Check sheet for the modelled part. Datum: model origin and axes. Units: mm. Face numbers are marked on the shaded views. A direction names the side the tool comes from. Coordinates: 2 decimals unless noted, no trailing zeros. Write each loop counter-clockwise with the first axis right and the second up, starting at its lowest first coordinate (ties: lowest second). Pieces come first, ordered by that corner, then holes. Notation, with made-up numbers: (-40, 72.5) -> (3, 72.5) arc R28 ccw to (3, 108.5) -> close; hole circle Ø11 at (85, 72). An arc over 180 degrees is marked (long way). One line per item, written item: value. Start each with the question number.
1) Sectioned sample at A-A on z = -88. Enter the section's corners in (x, y).
2) Sectioned sample at B-B on y = -4. Enter the section's corners in (x, z).
3) Set-up check for the marked faces 1, 2 and 3: record each of +Z, -Z, +X, -X, +Y, -Y from which the full face is reachable in a straight line by a thin tool's end or side.
4) Sectioned sample at D-D on y = -16. Enter the section's corners in (x, z).
5) Gauge pin test, flat ends, axial feed: P1, Ø4, axis at x = 48.5, z = -10, coming from the +Y side; P2, Ø9, axis at x = 44.5, y = -10, coming from the -Z side; P3, Ø1.5, axis at x = 31.5, z = -29, coming from the -Y side; P4, Ø9, axis at x = 34.81, z = -8, coming from the +Y side. Record the tip position at first contact, or that the pin passes through.
6) Draft check along Z on the marked faces 4, 5, 6 and 7. Enter one of: +Z half, -Z half, draft (parallel to the pull), parting line (faces both ways), or undercut.
7) Sectioned sample at C-C on z = -34. Enter the section's corners in (x, y).
8) Scan lines: line 1 along Z through (x, y) = (47, -9.5); line 2 along Z through (x, y) = (48, -13.5); line 3 along Z through (x, y) = (34, 7.25). Record each from-to range of solid material in increasing order. Write a range as [from, to].
```python
from build123d import *

# Parameters (mm, degrees)
SKETCH1_W                       = 52.809375
SKETCH1_H                       = 85
BOSS_EXTRUDE1_DEPTH             = 10
SPRING_PULLEY_CUTOUT_DEPTH      = 10
SPRING_PULLEY_CUTOUT_DEPTH_BACK = 11
SKETCH2_R                       = 24
BOSS_EXTRUDE4_DEPTH             = 23
SKETCH20_R                      = 2.75
CUT_EXTRUDE8_DEPTH              = 104.912607935
MOVE_START                      = -18
MOVE_FACE1_OUTLINE_W            = 23
MOVE_FACE1_OUTLINE_H            = 5
MOVE_FACE1_DEPTH                = 18
MOVE_FACE3_BY                   = 1
MOVE_FACE4_BY                   = 0.809375
FILLET4_R                       = 2
BOSS_EXTRUDE5_START             = -10
BOSS_EXTRUDE5_DEPTH             = 10
SKETCH38_R                      = 2.75
CUT_EXTRUDE9_DEPTH              = 118.140215502
CUT_EXTRUDE10_DEPTH             = 5


# Read off the part's stored shape, not the designer's step: Move Face1
with BuildPart() as part:
    # Sketch1 → Boss-Extrude1 (new body)
    with BuildSketch(Plane(origin=(0, 0, 0), x_dir=(1, 0, 0), z_dir=(0, 1, 0))):
        with Locations((26.4046875, 42.5)):
            Rectangle(SKETCH1_W, SKETCH1_H)
    extrude(amount=BOSS_EXTRUDE1_DEPTH)

    # Sketch2 → spring_pulley_cutout (cut, two sides: drawn at the far end of the back side and taken through both)
    with BuildSketch(Plane.ZY.offset(-18).offset(-SPRING_PULLEY_CUTOUT_DEPTH_BACK)):
        with Locations((-34, -18.5)):
            Circle(SKETCH2_R)
    extrude(amount=SPRING_PULLEY_CUTOUT_DEPTH + SPRING_PULLEY_CUTOUT_DEPTH_BACK, mode=Mode.SUBTRACT)

    # Sketch34 → Cut-Revolve1 (revolve, cut)
    with BuildSketch(Plane(origin=(16, 0, 0), x_dir=(0, 0, -1), z_dir=(1, 0, 0))):
        Polygon((16.798424815, -5.423086457), (21.139079438, 10.776457135), (24.036856917, 10), (23.001580737, 6.136296695), (21.069729084, 6.653934785), (17.764350642, -5.681905502), align=None)
    revolve(axis=Axis((16, -5.423086457, -16.798424815), (0, 0.9659258262890682, -0.2588190451025213)), mode=Mode.SUBTRACT)

    # Sketch36 → Cut-Revolve2 (revolve, cut)
    with BuildSketch(Plane(origin=(21, 0, 0), x_dir=(0, 0, -1), z_dir=(1, 0, 0)), mode=Mode.PRIVATE) as cut_revolve2_sk:
        Polygon((50.543888978, -2.968568117), (46.860920562, 10.776457135), (43.963143083, 10), (44.998419263, 6.136296695), (46.930270916, 6.653934785), (49.577963152, -3.227387162), align=None)
    revolve(cut_revolve2_sk.sketch.rotate(Axis((21, -2.968568117, -50.543888978), (0, 0.9659258262890665, 0.2588190451025275)), 180), axis=Axis((21, -2.968568117, -50.543888978), (0, 0.9659258262890665, 0.2588190451025275)), mode=Mode.SUBTRACT)

    # Sketch19 → Boss-Extrude4 (add)
    with BuildSketch(Plane.ZY.offset(-29.809375)):
        with BuildLine():
            Line((-68, -18), (-68, 0))
            Line((-68, 0), (0, 0))
            Line((0, 0), (0, -18))
            Line((0, -18), (-16.006945785, -18))
            ThreePointArc((-16.006945785, -18), (-34, -0.5), (-51.993054215, -18))
            Line((-51.993054215, -18), (-68, -18))
        make_face()
    extrude(amount=-BOSS_EXTRUDE4_DEPTH)

    # Sketch20 → Cut-Extrude8 (cut, through all)
    with BuildSketch(Plane(origin=(0, -18, 0), x_dir=(-1, 0, 0), z_dir=(0, -1, 0))):
        with Locations(Location((-47.809375, 8.003472892, 0), (0, 0, 90))):
            Circle(SKETCH20_R)
        with Locations(Location((-34.809375, 8.003472892, 0), (0, 0, 90))):
            Circle(SKETCH20_R)
        with Locations(Location((-47.809375, 59.996527108, 0), (0, 0, 90))):
            Circle(SKETCH20_R)
        with Locations(Location((-34.809375, 59.996527108, 0), (0, 0, 90))):
            Circle(SKETCH20_R)
    extrude(amount=-CUT_EXTRUDE8_DEPTH, mode=Mode.SUBTRACT)

    # Move Face1 outline → Move Face1 (add)
    with BuildSketch(Plane(origin=(0, 0, 0), x_dir=(1, 0, 0), z_dir=(0, 1, 0)).offset(MOVE_START)):
        with Locations((41.309375, 70.5)):
            Rectangle(MOVE_FACE1_OUTLINE_W, MOVE_FACE1_OUTLINE_H)
    extrude(amount=MOVE_FACE1_DEPTH)

    # Move Face3: a face moved inward by 1.0
    extrude(part.faces().sort_by_distance((8, 2.223147927, -34))[0], amount=MOVE_FACE3_BY, dir=(-1, 0, 0), mode=Mode.SUBTRACT)

    # Move Face4: a face moved inward by 0.809375
    extrude(part.faces().sort_by_distance((29, 2.223147927, -34))[0], amount=MOVE_FACE4_BY, dir=(1, 0, 0), mode=Mode.SUBTRACT)

    # Fillet4
    fillet4_edges = [part.edges().sort_by_distance(p)[0] for p in [
        (52.809375, -9, -73),
        (29.809375, -9, 0),
        (29.809375, -9, -73),
        (0, 5, -85),
        (52.809375, 5, -85),
        (52.809375, -4, 0),
        (0, 5, 0),
    ]]
    fillet(fillet4_edges, radius=FILLET4_R)

    # Sketch37 → Boss-Extrude5 (add)
    with BuildSketch(Plane.XZ.offset(BOSS_EXTRUDE5_START)):
        with BuildLine():
            Line((0, -83), (0, -101))
            ThreePointArc((0, -101), (0.585786438, -102.414213562), (2, -103))
            Line((2, -103), (50.809375, -103))
            ThreePointArc((50.809375, -103), (52.223588562, -102.414213562), (52.809375, -101))
            Line((52.809375, -101), (52.809375, -83))
            ThreePointArc((52.809375, -83), (52.223588562, -84.414213562), (50.809375, -85))
            Line((50.809375, -85), (2, -85))
            ThreePointArc((2, -85), (0.585786438, -84.414213562), (0, -83))
        make_face()
    extrude(amount=BOSS_EXTRUDE5_DEPTH)

    # Sketch38 → Cut-Extrude9 (cut, through all)
    with BuildSketch(Plane.XZ):
        with Locations(Location((12.5, -88, 0), (0, 0, 270))):
            Circle(SKETCH38_R)
        with Locations(Location((40.309375, -88, 0), (0, 0, 270))):
            Circle(SKETCH38_R)
    extrude(amount=-CUT_EXTRUDE9_DEPTH, mode=Mode.SUBTRACT)

    # Sketch39 → Cut-Extrude10 (cut)
    with BuildSketch(Plane(origin=(0, 10, 0), x_dir=(1, 0, 0), z_dir=(0, 1, 0))):
        Polygon((47.809375, 64.759666829), (43.684375, 62.378096968), (43.684375, 57.614957247), (47.809375, 55.233387387), (51.934375, 57.614957247), (51.934375, 62.378096968), align=None)
        Polygon((34.809375, 64.759666829), (30.684375, 62.378096968), (30.684375, 57.614957247), (34.809375, 55.233387387), (38.934375, 57.614957247), (38.934375, 62.378096968), align=None)
        Polygon((34.809375, 12.766612613), (30.684375, 10.385042753), (30.684375, 5.621903032), (34.809375, 3.240333171), (38.934375, 5.621903032), (38.934375, 10.385042753), align=None)
        Polygon((47.809375, 12.766612613), (43.684375, 10.385042753), (43.684375, 5.621903032), (47.809375, 3.240333171), (51.934375, 5.621903032), (51.934375, 10.385042753), align=None)
    extrude(amount=-CUT_EXTRUDE10_DEPTH, mode=Mode.SUBTRACT)


solid = part.part
```
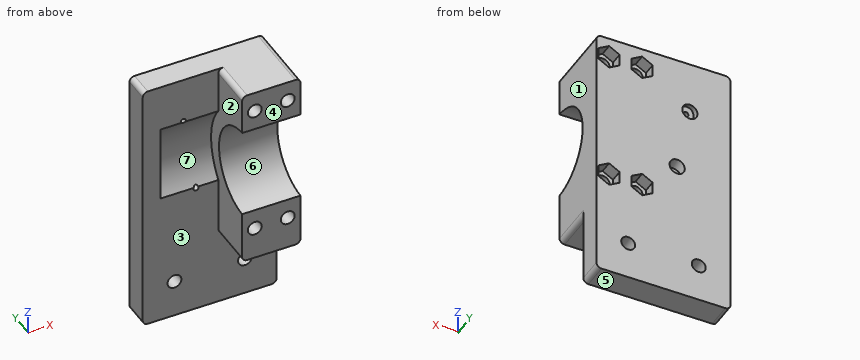
Answers:
1. outline: (0, 0) -> (9.75, 0) -> (9.75, 10) -> (0, 10) -> close; (15.25, 0) -> (37.56, 0) -> (37.56, 10) -> (15.25, 10) -> close; (43.06, 0) -> (52.81, 0) -> (52.81, 10) -> (43.06, 10) -> close
2. outline: (29.81, -71) arc R2 ccw to (31.81, -73) -> (50.81, -73) arc R2 ccw to (52.81, -71) -> (52.81, -44.67) -> (29.81, -44.67) -> close; (29.81, -23.33) -> (52.81, -23.33) -> (52.81, -2) arc R2 ccw to (50.81, 0) -> (31.81, 0) arc R2 ccw to (29.81, -2) -> close; hole circle Ø5.5 at (34.81, -60); hole circle Ø5.5 at (34.81, -8); hole circle Ø5.5 at (47.81, -60); hole circle Ø5.5 at (47.81, -8)
3. face 1: +Z, -Z, +X, +Y, -Y
3. face 2: -Y
3. face 3: -Z, -X, -Y
4. outline: (29.81, -71) arc R2 ccw to (31.81, -73) -> (50.81, -73) arc R2 ccw to (52.81, -71) -> (52.81, -51.83) -> (29.81, -51.83) -> close; (29.81, -16.17) -> (52.81, -16.17) -> (52.81, -2) arc R2 ccw to (50.81, 0) -> (31.81, 0) arc R2 ccw to (29.81, -2) -> close; hole circle Ø5.5 at (34.81, -60); hole circle Ø5.5 at (34.81, -8); hole circle Ø5.5 at (47.81, -60); hole circle Ø5.5 at (47.81, -8)
5. P1: stops at y = 5
5. P2: stops at z = -73
5. P3: stops at y = -1.44
5. P4: stops at y = 10
6. face 4: draft
6. face 5: -Z half
6. face 6: undercut
6. face 7: undercut
7. outline: (0, 0) -> (7, 0) -> (7, 5.5) -> (29.81, 5.5) -> (29.81, -0.5) -> (52.81, -0.5) -> (52.81, 10) -> (0, 10) -> close
8. line 1: z = [-73, -62.62], [-57.37, -49.59], [-18.41, -10.63], [-5.38, 0]
8. line 2: z = [-73, -62.74], [-57.25, -51.29], [-16.71, -10.75], [-5.26, 0]
8. line 3: z = [-103, -64.29], [-55.7, -12.3], [-3.71, 0]
